from build123d import *

# Parameters (mm, degrees)
F0_R     = 74.93
F0_R_2   = 28.5
F1_DEPTH = 30


with BuildPart() as f1:
    # F0 (on Top) → F1 (new body)
    with BuildSketch(Plane.XY):
        Circle(F0_R)
        with BuildLine():
            ThreePointArc((5.98919, 49.64), (35.355339, 35.355339), (49.64, 5.98919))
            ThreePointArc((49.64, 5.98919), (54.113393, 4.368066), (56, 0))
            ThreePointArc((56, 0), (54.113393, -4.368066), (49.64, -5.98919))
            ThreePointArc((49.64, -5.98919), (35.355339, -35.355339), (5.98919, -49.64))
            ThreePointArc((5.98919, -49.64), (5.997297, -49.819919), (6, -50))
            ThreePointArc((6, -50), (-0.180081, -55.997297), (-5.98919, -49.64))
            ThreePointArc((-5.98919, -49.64), (-35.355339, -35.355339), (-49.64, -5.98919))
            ThreePointArc((-49.64, -5.98919), (-56, 0), (-49.64, 5.98919))
            ThreePointArc((-49.64, 5.98919), (-35.355339, 35.355339), (-5.98919, 49.64))
            ThreePointArc((-5.98919, 49.64), (-0.180081, 55.997297), (6, 50))
            ThreePointArc((6, 50), (5.997297, 49.819919), (5.98919, 49.64))
        make_face(mode=Mode.SUBTRACT)
        with BuildLine():
            ThreePointArc((49.64, -5.98919), (44, 0), (49.64, 5.98919))
            ThreePointArc((49.64, 5.98919), (35.355339, 35.355339), (5.98919, 49.64))
            ThreePointArc((5.98919, 49.64), (0, 44), (-5.98919, 49.64))
            ThreePointArc((-5.98919, 49.64), (-35.355339, 35.355339), (-49.64, 5.98919))
            ThreePointArc((-49.64, 5.98919), (-45.631934, 4.113393), (-44, 0))
            ThreePointArc((-44, 0), (-45.631934, -4.113393), (-49.64, -5.98919))
            ThreePointArc((-49.64, -5.98919), (-35.355339, -35.355339), (-5.98919, -49.64))
            ThreePointArc((-5.98919, -49.64), (0, -44), (5.98919, -49.64))
            ThreePointArc((5.98919, -49.64), (35.355339, -35.355339), (49.64, -5.98919))
        make_face()
        Circle(F0_R_2, mode=Mode.SUBTRACT)
    extrude(amount=F1_DEPTH)


solid = f1.part
The model under review builds one solid part; all positions refer to its coordinate system, in mm. Give positions to 0.01 mm unless a question says otherwise; leave off trailing zeros. Write each loop counter-clockwise with the first axis right and the second up, starting at its lowest first coordinate (ties: lowest second). Pieces come first, ordered by that corner, then holes.
1. Add section A-A, the plane x = 0. Write out the cut boundary in (y, z).
2. Draft analysis for pull direction Y (two halves, no side actions). For faces 1 (the flat face through (-1, -32, 30)), 2 (the cylindrical face through (-59.462, -45.594, 14.79)), 3 (the cylindrical face through (26.327, -10.916, 14.79)), state which applies: +Y half, -Y half, draft (parallel to the pull), parting line (faces both ways), or undercut.
3. Wall thickness on L1, parallel to Y at x = 0, z = 19.75; L2, parallel to X at y = 54.5, z = 10; L3, parallel to X at y = -51, z = 4: over which ranges is each line inside the solid? List them lowest first.
4. Add section B-B, the plane z = 5.25. Write out the cut boundary in (x, y), plus the area to 3 significant figures.
5. Add section C-C, the plane y = 23.5. Write out the cut boundary in (x, z), plus the area to 3 significant figures.
6. Add section D-D, the plane x = -20.5. Write out the cut boundary in (y, z).
7. For P1, Ø2, axis at y = 16, z = 12.5, coming from the -X side; P2, Ø10, axis at x = 19, y = -7.5, coming from the +Z side; P3, Ø10, axis at x = -58.5, z = 15.5, coming from the -Y side; P4, Ø10, axis at x = 42.5, z = 8, coming from the -Y side, all flat-tipped, find the tip position at first contact; note any pin that passes through.
Worked answers:
1. outline: (-74.93, 0) - (-56, 0) - (-56, 30) - (-74.93, 30) - close; (-44, 0) - (-28.5, 0) - (-28.5, 30) - (-44, 30) - close; (28.5, 0) - (44, 0) - (44, 30) - (28.5, 30) - close; (56, 0) - (74.93, 0) - (74.93, 30) - (56, 30) - close
2. face 1: draft
2. face 2: parting line
2. face 3: undercut
3. L1: y = -74.93 to -56, -44 to -28.5, 28.5 to 44, 56 to 74.93
3. L2: x = -51.42 to -3.97, 3.97 to 51.42
3. L3: x = -54.9 to -5.92, 5.92 to 54.9
4. outline: circle Ø149.86 at (0, 0); hole (-49.64, -5.99) arc R6 ccw to (-44, 0) arc R6 ccw to (-49.64, 5.99) arc R6 ccw (long way) to start; hole circle Ø57 at (0, 0); hole (5.99, -49.64) arc R6 ccw (long way) to (6, -50) arc R6 ccw to start; hole (5.99, 49.64) arc R6 ccw to (6, 50) arc R6 ccw (long way) to start; hole (49.64, -5.99) arc R6 ccw to (56, 0) arc R6 ccw to (49.64, 5.99) arc R6 ccw to start
4. area: 14,600 mm2
5. outline: (-71.15, 0) - (-16.12, 0) - (-16.12, 30) - (-71.15, 30) - close; (16.12, 0) - (71.15, 0) - (71.15, 30) - (16.12, 30) - close
5. area: 3,300 mm2
6. outline: (-72.07, 0) - (-19.8, 0) - (-19.8, 30) - (-72.07, 30) - close; (19.8, 0) - (72.07, 0) - (72.07, 30) - (19.8, 30) - close
7. P1: stops at x = -73.41
7. P2: passes through
7. P3: stops at y = -52.46
7. P4: stops at y = -64.87
